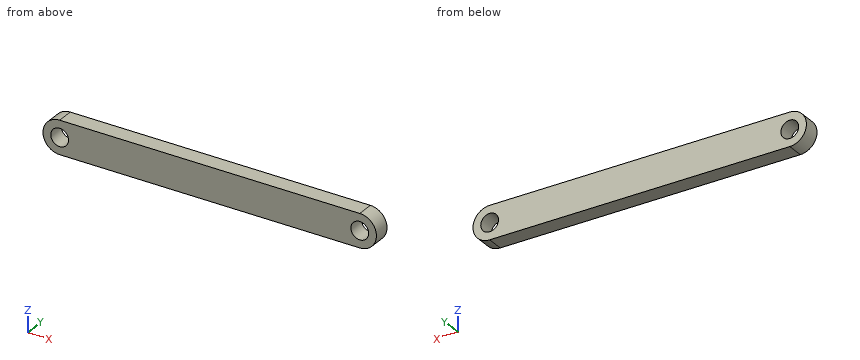
from build123d import *

# Parameters (mm, degrees)
EXTRUDE_1_DEPTH     = 3
SKETCH_2_R          = 1.6
CUT_EXTRUDE_1_DEPTH = 4


with BuildPart() as part:
    # 草图1 → 凸台-拉伸1 (new body)
    with BuildSketch(Plane(origin=(0, 0, 0), x_dir=(1, 0, 0), z_dir=(0, 1, 0))):
        with BuildLine():
            Line((-54, -3), (0, -3))
            ThreePointArc((0, -3), (3, 0), (0, 3))
            Line((0, 3), (-54, 3))
            ThreePointArc((-54, 3), (-57, 0), (-54, -3))
        make_face()
    extrude(amount=EXTRUDE_1_DEPTH)

    # 草图2 → 切除-拉伸1 (cut, through all)
    with BuildSketch(Plane(origin=(0, 3, 0), x_dir=(1, 0, 0), z_dir=(0, 1, 0))):
        with Locations((-54, 0)):
            Circle(SKETCH_2_R)
        Circle(SKETCH_2_R)
    extrude(amount=-CUT_EXTRUDE_1_DEPTH, mode=Mode.SUBTRACT)


solid = part.part
CAD build for the part. Positions are in the model's coordinates, mm. Coordinates: 2 decimals unless noted, no trailing zeros. Loops run counter-clockwise (first coordinate to the right, second up) from the corner with the lowest first, then second, coordinate; pieces in that order, holes last. Notation, with made-up numbers: (-21.5, 79) - (-7.5, 79) arc R13 ccw to (-7.5, 88) - close; hole circle Ø6 at (63, 31). An arc over 180 degrees is marked (long way). Use one line per item in the form item = value. Start each with the question number.
1) Band-saw the part on C-C (z = 2.45). Give the cut face in (x, y).
2) Band-saw the part on B-B (y = 2.2). Give the cut face in (x, z), and give its area (3 significant figures).
3) Flat gauge pin, fed straight in: pin 1 (1.9 mm diameter, centred on x = 0, z = 0, fed in from -Y). Where does the tip first touch, or does it go through?
4) Band-saw the part on A-A (z = -0.8). Give the cut face in (x, y).
5) Drill centre lines: L1, parallel to X at y = 1.5, z = 0; L2, parallel to Z at x = -54, y = 1; L3, parallel to X at y = 2.8, z = -0.9. Where is each one in solid material? Low to high. Write a range as from..to.
Check values:
q1.outline = (-55.73, 0) - (1.73, 0) - (1.73, 3) - (-55.73, 3) - close
q2.outline = (-54, -3) - (0, -3) arc R3 ccw to (0, 3) - (-54, 3) arc R3 ccw to start; hole circle Ø3.2 at (-54, 0); hole circle Ø3.2 at (0, 0)
q2.area = 336 mm2
q3.pin_1 = through
q4.outline = (-56.89, 0) - (-55.39, 0) - (-55.39, 3) - (-56.89, 3) - close; (-52.61, 0) - (-1.39, 0) - (-1.39, 3) - (-52.61, 3) - close; (1.39, 0) - (2.89, 0) - (2.89, 3) - (1.39, 3) - close
q5.L1 = -57..-55.6, -52.4..-1.6, 1.6..3
q5.L2 = -3..-1.6, 1.6..3
q5.L3 = -56.86..-55.32, -52.68..-1.32, 1.32..2.86
